Geometry check sheet. Reference: the model listing, model coordinates, mm. Face numbers are marked on the shaded views. A direction names the side the tool comes from. Round coordinates to 2 decimals unless told otherwise and drop trailing zeros. Order: outer loops, then holes, each group sorted by start corner. A loop starts at its lowest first (then second) coordinate and runs counter-clockwise, first axis right, second up. Notation, with made-up numbers: (1, 79) - (36, 79) arc R9 ccw to (36, 93) - close; hole circle Ø10 at (65.5, 39.5). An arc over 180 degrees is marked (long way). One line per question, with ' | ' between items. Start each with the question number.
Q1. Tool access check on the marked faces 1 and 2. Record the directions out of +Z, -Z, +X, -X, +Y, -Y that give a thin tool (end or side, any length) a straight path to the whole face; none if there is none.
Q2. Sectioned sample at A-A, the plane x = 0. Enter the section's corners in (y, z), then the cut area to 3 significant figures.
Q3. Material ranges on line 1 along Y through (x, z) = (-43, -41.5); line 2 along Y through (x, z) = (0, -31); line 3 along Y through (x, z) = (0, 5), recorded low to high.
Q4. Sectioned sample at B-B, the plane y = -116. Enter the section's corners in (x, z), then the cut area to 3 significant figures.
Q5. Sectioned sample at C-C, the plane y = -90.5. Enter the section's corners in (x, z).
Q6. Gauge pin test, flat ends, axial feed: P1, Ø2, axis at y = -42.5, z = -13.5, coming from the -X side; P2, Ø19, axis at x = 0, y = -36.62, coming from the +Z side; P3, Ø3, axis at x = -49, z = -14.5, coming from the +Y side; P4, Ø9.5, axis at x = 0, y = -36.62, coming from the -Z side. Record the tip position at first contact, or that the pin passes through.
```python
from build123d import *

# Parameters (mm, degrees)
F2_SIZE2      = 10
F2_SIZE       = 10
F3_SIZE2      = 10
F3_SIZE       = 10
F4_R          = 6
F5_DEPTH      = 80.6255635247
F5_DEPTH_BACK = 49.3764364753


with BuildPart() as f1:
    # F0 (on Right) → F1 (revolve)
    with BuildSketch(Plane.YZ):
        Polygon((-138.6194518108, 49.3754364753), (-138.6194518108, -15.6245635247), (-18.6194518108, -15.6245635247), (-18.6194518108, 9.3754364753), (-108.6194518108, 9.3754364753), (-108.6194518108, 49.3754364753), align=None)
    revolve(axis=Axis((0, -78.6194518108, -15.6245635247), (0, 1, 0)))

    # F2
    f2_edges = [f1.edges().sort_by_distance(p)[0] for p in [
        (0, -18.619452, -40.624564),
    ]]
    chamfer(f2_edges, length=F2_SIZE, length2=F2_SIZE2)

    # F3
    f3_edges = [f1.edges().sort_by_distance(p)[0] for p in [
        (0, -138.619452, -80.624564),
    ]]
    chamfer(f3_edges, length=F3_SIZE, length2=F3_SIZE2)

    # F4 (on Top) → F5 (cut, two sides)
    with BuildSketch(Plane.XY) as f5_sk:
        with Locations((0, -36.6194518108)):
            Circle(F4_R)
    extrude(amount=-F5_DEPTH, mode=Mode.SUBTRACT)
    extrude(f5_sk.sketch, amount=F5_DEPTH_BACK, mode=Mode.SUBTRACT)


solid = f1.part
```
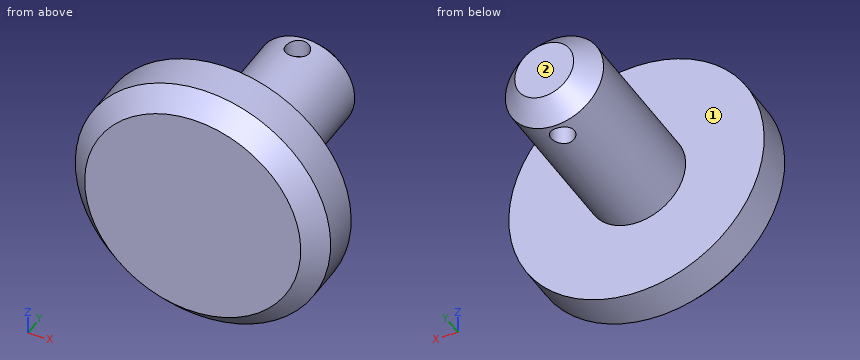
Determined:
1) face 1: +Y | face 2: +Z, -Z, +X, -X, +Y
2) outline: (-138.62, -70.62) - (-128.62, -80.62) - (-108.62, -80.62) - (-108.62, -40.62) - (-42.62, -40.62) - (-42.62, 9.38) - (-108.62, 9.38) - (-108.62, 49.38) - (-128.62, 49.38) - (-138.62, 39.38) - close; (-30.62, -40.62) - (-28.62, -40.62) - (-18.62, -30.62) - (-18.62, -0.62) - (-28.62, 9.38) - (-30.62, 9.38) - close | area: 7,600 mm2
3) line 1: y = -138.62 to -108.62 | line 2: y = -138.62 to -42.62, -30.62 to -18.99 | line 3: y = -138.62 to -42.62, -30.62 to -24.24
4) outline: circle Ø130 at (0, -15.62) | area: 13,300 mm2
5) outline: circle Ø50 at (0, -15.62)
6) P1: stops at x = -24.97 | P2: stops at z = 9.38 | P3: stops at y = -108.62 | P4: passes through
